Here's how the part is built. I have some questions about the finished solid (model axes, mm). A direction names the side the tool comes from. Round coordinates to 2 decimals unless told otherwise and drop trailing zeros. Write each loop counter-clockwise with the first axis right and the second up, starting at its lowest first coordinate (ties: lowest second). Pieces come first, ordered by that corner, then holes. Notation, with made-up numbers: (-7.5, -15.5) -> (1.5, -15.5) arc R34 ccw to (1.5, 18.5) -> close; hole circle Ø6 at (61.25, 11). An arc over 180 degrees is marked (long way). Answer in a Markdown table with one row per item.
from build123d import *

# Parameters (mm, degrees)
ESQUISSE1_W        = 53.8
ESQUISSE1_H        = 25.15
BOSS_EXTRU_1_DEPTH = 5.2
ESQUISSE2_W        = 4.75
ESQUISSE2_H        = 25.15
BOSS_EXTRU_2_DEPTH = 12.1
BOSS_EXTRU_3_START = -4.75
BOSS_EXTRU_3_DEPTH = 4.75
ESQUISSE4_W        = 4.7
ESQUISSE4_H        = 25.15
BOSS_EXTRU_4_DEPTH = 12.1
BOSS_EXTRU_5_START = -4.7
BOSS_EXTRU_5_DEPTH = 4.7


with BuildPart() as part:
    # Esquisse1 → Boss.-Extru.1 (new body)
    with BuildSketch(Plane(origin=(0, 0, 0), x_dir=(1, 0, 0), z_dir=(0, 1, 0))):
        Rectangle(ESQUISSE1_W, ESQUISSE1_H)
    extrude(amount=BOSS_EXTRU_1_DEPTH)

    # Esquisse2 → Boss.-Extru.2 (add)
    with BuildSketch(Plane(origin=(0, 5.2, 0), x_dir=(1, 0, 0), z_dir=(0, 1, 0))):
        with Locations((-24.525, 0)):
            Rectangle(ESQUISSE2_W, ESQUISSE2_H)
    extrude(amount=BOSS_EXTRU_2_DEPTH)

    # Esquisse3 → Boss.-Extru.3 (add)
    with BuildSketch(Plane.ZY.offset(26.9).offset(BOSS_EXTRU_3_START)):
        with BuildLine():
            Line((12.575, 17.3), (-12.575, 17.3))
            ThreePointArc((-12.575, 17.3), (0, 29.875), (12.575, 17.3))
        make_face()
    extrude(amount=BOSS_EXTRU_3_DEPTH)

    # Esquisse4 → Boss.-Extru.4 (add)
    with BuildSketch(Plane(origin=(0, 5.2, 0), x_dir=(1, 0, 0), z_dir=(0, 1, 0))):
        with Locations((24.55, 0)):
            Rectangle(ESQUISSE4_W, ESQUISSE4_H)
    extrude(amount=BOSS_EXTRU_4_DEPTH)

    # Esquisse5 → Boss.-Extru.5 (add)
    with BuildSketch(Plane(origin=(26.9, 0, 0), x_dir=(0, 0, -1), z_dir=(1, 0, 0)).offset(BOSS_EXTRU_5_START)):
        with BuildLine():
            Line((12.575, 17.3), (-12.575, 17.3))
            ThreePointArc((-12.575, 17.3), (0, 29.875), (12.575, 17.3))
        make_face()
    extrude(amount=BOSS_EXTRU_5_DEPTH)


solid = part.part
1) I want a section at B-B, the plane z = 0. List the corners of the cut face in (x, y) for me (3 decimals), and give its area (3 significant figures).
Response:
| item | result |
|---|---|
| outline | (-26.9, 0) -> (26.9, 0) -> (26.9, 29.875) -> (22.2, 29.875) -> (22.2, 5.2) -> (-22.15, 5.2) -> (-22.15, 29.875) -> (-26.9, 29.875) -> close |
| area | 513 mm^2 |
2) I need wall thicknesses on line 1 (X direction, y = 18.5, z = 3.75); line 2 (Y direction, x = 17.5, z = -3). Which ranges of each line are inside material? Lowest first, please. Write a range as [from, to].
Response:
| item | result |
|---|---|
| line 1 | x = [-26.9, -22.15], [22.2, 26.9] |
| line 2 | y = [0, 5.2] |
3) Which directions (+Z, -Z, +X, -X, +Y, -Y) give clear straight access to the entire face, cutting with the end or side of a thin tool? Please do faces 4 (the face through (0, 0, 0)), 5 (the face through (22.2, 18, 0)).
Response:
| item | result |
|---|---|
| face 4 | +Z, -Z, +X, -X, -Y |
| face 5 | +Z, -Z, +Y |
4) For pin 1 (5 mm diameter, centred on x = -7.5, z = -8.5, fed in from +Y), with a flat end and sliding along its axis, tell me the tip position at first contact or that it passes through.
Response:
| item | result |
|---|---|
| pin 1 | stops at y = 5.2 |
5) I want a section at A-A, the plane y = 7.25. List the corners of the cut face in (x, z) for me (3 decimals).
Response:
| item | result |
|---|---|
| outline | (-26.9, -12.575) -> (-22.15, -12.575) -> (-22.15, 12.575) -> (-26.9, 12.575) -> close; (22.2, -12.575) -> (26.9, -12.575) -> (26.9, 12.575) -> (22.2, 12.575) -> close |
6) I want a section at D-D, the plane x = 1.5. List the corners of the cut face in (y, z) for me (3 decimals), and give its area (3 significant figures).
Response:
| item | result |
|---|---|
| outline | (0, -12.575) -> (5.2, -12.575) -> (5.2, 12.575) -> (0, 12.575) -> close |
| area | 131 mm^2 |
7) I want a section at C-C, the plane y = 21. List the corners of the cut face in (x, z) for me.
Response:
| item | result |
|---|---|
| outline | (-26.9, -12.02) -> (-22.15, -12.02) -> (-22.15, 12.02) -> (-26.9, 12.02) -> close; (22.2, -12.02) -> (26.9, -12.02) -> (26.9, 12.02) -> (22.2, 12.02) -> close |
8) We'd pull the mould along X, two halves only. Please class faces 1 (the face through (26.9, 15, 0)), 2 (the face through (0, 5.2, 0)), 3 (the face through (0, 5, -12.575)): +X half, -X half, draft (parallel to the pull), parting line (faces both ways), or undercut.
Response:
| item | result |
|---|---|
| face 1 | +X half |
| face 2 | undercut |
| face 3 | draft |
